Input: dimensioned drawing with shaded views. Units: mm. Origin: part minimum x, y, z. Give positions to 0.01 mm unless a question says otherwise; leave off trailing zeros. Write each loop counter-clockwise with the first axis right and the second up, starting at its lowest first coordinate (ties: lowest second). Pieces come first, ordered by that corner, then holes.
Q1. Line query: line 1 (X direction, y = 33, z = 11.5) (1 decimal); line 2 (X direction, y = 51, z = 8.5); line 3 (Z direction, x = 8, y = 48). Output: solid intervals per line, ascending.
Q2. Pin query (flat end, axial travel): pin 1 Ø4 at (x, y) = (6, 7.5) entering from -Z (1 decimal); pin 2 Ø3 at (y, z) = (22.5, 4) entering from +X; pin 3 Ø2 at (x, z) = (3.5, 7.5) entering from -Y. Return the tip coordinate at first contact, or that it passes through.
Q3. Section A-A (y = 51). Return the cut outline in (x, z).
Q4. Mould query, pull axis Y, two halves, no side actions, for the marked faces 1, 2 and 3. Classes: +Y half, -Y half, draft (parallel to the pull), parting line (faces both ways), or undercut.
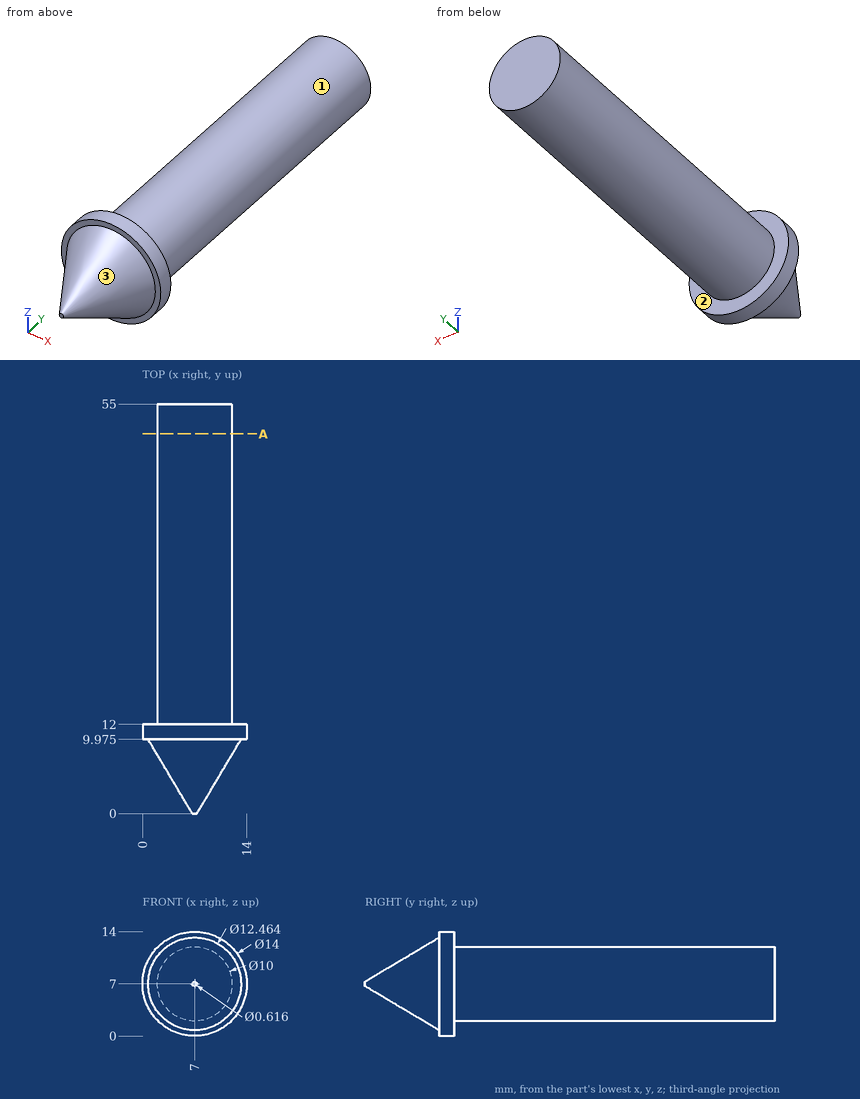
Computed:
1. line 1: x = 4.8 to 9.2
1. line 2: x = 2.23 to 11.77
1. line 3: z = 2.1 to 11.9
2. pin 1: stops at z = 1.1
2. pin 2: stops at x = 11.77
2. pin 3: stops at y = 3.75
3. outline: circle Ø10 at (7, 7)
4. face 1: draft
4. face 2: +Y half
4. face 3: -Y half
